For this review, take the finished solid that the model builds, in its own axes (mm). Face numbers are marked on the shaded views. Coordinates: 2 decimals unless noted, no trailing zeros. Order: outer loops, then holes, each group sorted by start corner. A loop starts at its lowest first (then second) coordinate and runs counter-clockwise, first axis right, second up.
from build123d import *

# Parameters (mm, degrees)
F2_R     = 2.5
F3_DEPTH = 35.001
F4_R     = 5
F4_R_2   = 2.5
F5_DEPTH = 20


with BuildPart() as f1:
    # F0 (on Right) → F1 (revolve)
    with BuildSketch(Plane.YZ):
        Polygon((25, 0), (0, 0), (0, -35), (10, -35), align=None)
    revolve(axis=Axis((0, 0, -17.5), (0, 0, 1)))

    # F2 (on face) → F3 (cut, through all)
    with BuildSketch(Plane.XY):
        Circle(F2_R)
    extrude(amount=-F3_DEPTH, mode=Mode.SUBTRACT)

    # F4 (on face) → F5 (cut)
    with BuildSketch(Plane(origin=(0, 0, -35), x_dir=(1, 0, 0), z_dir=(0, 0, -1))):
        Circle(F4_R)
        Circle(F4_R_2, mode=Mode.SUBTRACT)
    extrude(amount=-F5_DEPTH, mode=Mode.SUBTRACT)


solid = f1.part
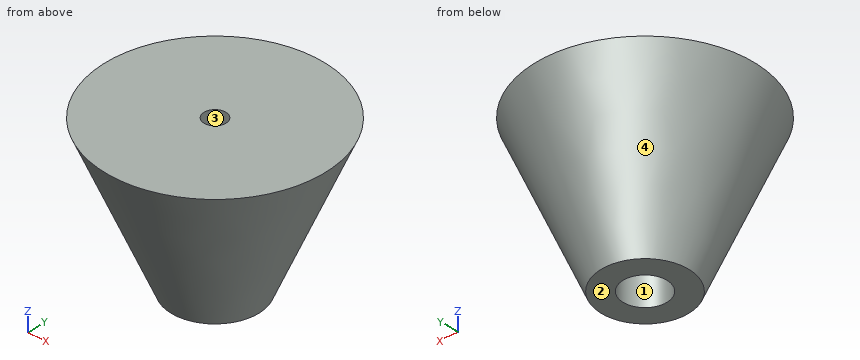
1. Take a section at A-A, the plane y = 0. Give the boundary of the cut face in (x, z).
Answer below:
outline: (-25, 0) - (-10, -35) - (-5, -35) - (-5, -15) - (-2.5, -15) - (-2.5, 0) - close; (2.5, -15) - (5, -15) - (5, -35) - (10, -35) - (25, 0) - (2.5, 0) - close
2. Take a section at D-D, the plane z = -30. Give the boundary of the cut face in (x, y).
Answer below:
outline: circle Ø24.29 at (0, 0); hole circle Ø10 at (0, 0)
3. Take a section at C-C, the plane z = -20.5. Give the boundary of the cut face in (x, y), plus the area to 3 significant figures.
Answer below:
outline: circle Ø32.43 at (0, 0); hole circle Ø10 at (0, 0)
area: 747 mm2
4. To check wall thickness, follow L1, parallel to Y at x = 0, z = -4; L2, parallel to X at y = 0, z = -24; L3, parallel to Y at x = 0, z = -28. State the ranges of each line that lie inside material, in increasing order.
Answer below:
L1: y = -23.29 to -2.5, 2.5 to 23.29
L2: x = -14.71 to -5, 5 to 14.71
L3: y = -13 to -5, 5 to 13
5. The part is to be moulded in two halves that separate along X. For the marked faces 1, 2, 3 and 4, say which applies: +X half, -X half, draft (parallel to the pull), parting line (faces both ways), or undercut.
Answer below:
face 1: undercut
face 2: draft
face 3: undercut
face 4: parting line
6. Clearance check with flat-ended pins moving along their axes: pin 1 Ø1 at (y, z) = (-4.5, -6) entering from -X; pin 2 Ø5 at (x, y) = (-15, 4) entering from -Z; pin 3 Ø5 at (x, z) = (12, -22.5) entering from -Y. State where each tip first meets the part, or that it passes through.
Answer below:
pin 1: stops at x = -22.21
pin 2: stops at z = -27.94
pin 3: stops at y = -12.49
